Input: part model. Units: mm. Frame: model coordinates. Face numbers are marked on the shaded views. A direction names the side the tool comes from. Give positions to 0.01 mm unless a question says otherwise; leave off trailing zeros. Loops run counter-clockwise (first coordinate to the right, second up) from the corner with the lowest first, then second, coordinate; pieces in that order, holes last. Notation, with made-up numbers: (54, -26) -> (97, -26) arc R29 cw to (97, 3) -> close; hole circle Ø4 at (-11.5, 17). An arc over 180 degrees is marked (long way). Use CSV: the item, a comma, the result in double quotes.
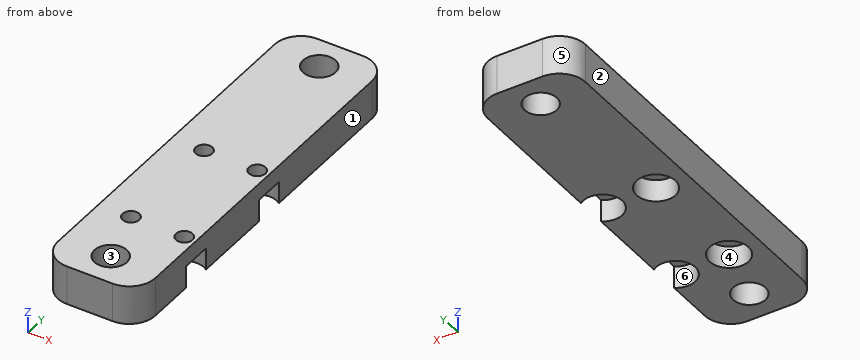
```python
from build123d import *

# Parameters (mm, degrees)
SKETCH1_W                                      = 19.05
SKETCH1_H                                      = 76.2
BOSS_EXTRUDE1_DEPTH                            = 7.62
F_1_4_0_25_DIAMETER_HOLE1_D                    = 6.35
F_1_4_0_25_DIAMETER_HOLE1_DEPTH                = 25.4
F_1_4_0_25_DIAMETER_HOLE1_TIP                  = 1.907732465
CBORE_FOR_4_SOCKET_HEAD_CAP_SCREW5_D           = 3.2639
CBORE_FOR_4_SOCKET_HEAD_CAP_SCREW5_CBORE_D     = 7.62
CBORE_FOR_4_SOCKET_HEAD_CAP_SCREW5_CBORE_DEPTH = 4.318
FILLET1_R                                      = 5.08


with BuildPart() as part:
    # Sketch1 → Boss-Extrude1 (new body)
    with BuildSketch(Plane.XY):
        with Locations((-4.445, -9.525)):
            Rectangle(SKETCH1_W, SKETCH1_H)
    extrude(amount=BOSS_EXTRUDE1_DEPTH)

    # 1/4 (0.25) Diameter Hole1
    with Locations(Plane.XY.offset(7.62)):
        with Locations((-4.445, 22.225), (-4.445, -41.275)):
            Hole(F_1_4_0_25_DIAMETER_HOLE1_D / 2, depth=F_1_4_0_25_DIAMETER_HOLE1_DEPTH)
            with Locations((0, 0, -(F_1_4_0_25_DIAMETER_HOLE1_DEPTH + F_1_4_0_25_DIAMETER_HOLE1_TIP / 2))):  # 118° drill point
                Cone(0, F_1_4_0_25_DIAMETER_HOLE1_D / 2, F_1_4_0_25_DIAMETER_HOLE1_TIP, mode=Mode.SUBTRACT)

    # CBORE for #4 Socket Head Cap Screw5 (through all)
    with Locations(Plane(origin=(-2.017261163, -3.813643011, 0), x_dir=(1, 0, 0), z_dir=(0, 0, -1))):
        with Locations((-5.602738837, 4.123856989), (-5.602738837, 26.348856989), (4.811261163, 26.348856989), (4.811261163, 4.123856989)):
            CounterBoreHole(CBORE_FOR_4_SOCKET_HEAD_CAP_SCREW5_D / 2, CBORE_FOR_4_SOCKET_HEAD_CAP_SCREW5_CBORE_D / 2, CBORE_FOR_4_SOCKET_HEAD_CAP_SCREW5_CBORE_DEPTH)

    # Fillet1
    fillet1_edges = [part.edges().sort_by_distance(p)[0] for p in [
        (-13.97, 28.575, 3.81),
        (5.08, 28.575, 3.81),
        (5.08, -47.625, 3.81),
        (-13.97, -47.625, 3.81),
    ]]
    fillet(fillet1_edges, radius=FILLET1_R)


solid = part.part
```
1) Section query A-A (y = -39). Return loops of the section in (x, z).
From the geometry:
outline,"(-13.97, 0) -> (-6.66, 0) -> (-6.66, 7.62) -> (-13.97, 7.62) -> close; (-2.23, 0) -> (5.08, 0) -> (5.08, 7.62) -> (-2.23, 7.62) -> close"
2) Section query B-B (z = 1). Give the number of separate pieces and of enclosed holes in the cut face, then the cut area to 3 significant figures.
From the geometry:
separate pieces,"1"
enclosed holes,"4"
area,"1,200 mm^2"
3) Reachability of the marked faces 5 and 6 from +Z, -Z, +X, -X, +Y, -Y: full face, straight path, thin tool, end or side. Return the list, or none.
From the geometry:
face 5,"+Z, -Z, -X, +Y"
face 6,"-Z"
4) Ray query, line 1 (X direction, y = -4.5, z = 2.5); line 2 (Y direction, x = -6.75, z = 1) (3 decimals); line 3 (Y direction, x = -6, z = 3.25) (3 decimals). Return the intervals inside material, ascending.
From the geometry:
line 1,"x = -13.97 to -9.26, -5.98 to 1.15, 4.44 to 5.08"
line 2,"y = -47.625 to -43.458, -39.092 to -33.872, -26.453 to -11.647, -4.228 to 20.042, 24.408 to 28.575"
line 3,"y = -47.625 to -44.043, -38.507 to -33.611, -26.714 to -11.386, -4.489 to 19.457, 24.993 to 28.575"
5) Mould query, pull axis X, two halves, no side actions, for the marked faces 1, 2, 3 and 4. Classes: pulls with the +X half, pulls with the -X half, needs draft (parallel to the pull), parting line crosses it, or undercut.
From the geometry:
face 1,"pulls with the +X half"
face 2,"pulls with the -X half"
face 3,"undercut"
face 4,"undercut"
6) Contact query for flat-ended pins moving along their axis: pin 1 (3 mm diameter, centred on x = 1.5, y = -8.5, fed in from -Z); pin 2 (3 mm diameter, centred on x = -7.62, y = -7.94, fed in from +Z). Output: stop coordinate, or through.
From the geometry:
pin 1,"stops at z = 4.32"
pin 2,"passes through"
